```python
from build123d import *

# Parameters (mm, degrees)
BOSS_EXTRUDE1_DEPTH = 5.842
FILLET1_R           = 3.175


with BuildPart() as part:
    # Sketch1 → Boss-Extrude1 (new body)
    with BuildSketch(Plane(origin=(0, 0, 0), x_dir=(1, 0, 0), z_dir=(0, 1, 0))):
        Polygon((25.4, -34.925), (17.895454545, -34.925), (6.35, -19.05), (-6.35, -19.05), (-17.895454545, -34.925), (-25.4, -34.925), (-25.4, -31.75), (-31.242, -31.75), (-31.242, -19.05), (-25.4, -19.05), (-25.4, -14.4526), (-19.05, -14.4526), (-19.05, -15.748), (-15.875, -15.748), (-15.875, -14.4526), (-11.692, -14.4526), (-11.692, -10.9474), (-15.875, -10.9474), (-15.875, -9.652), (-19.05, -9.652), (-19.05, -10.9474), (-25.4, -10.9474), (-25.4, -6.35), (-31.242, -6.35), (-31.242, 6.35), (-25.4, 6.35), (-25.4, 10.9474), (-19.05, 10.9474), (-19.05, 9.652), (-15.875, 9.652), (-15.875, 10.9474), (-11.692, 10.9474), (-11.692, 14.4526), (-15.875, 14.4526), (-15.875, 15.748), (-19.05, 15.748), (-19.05, 14.4526), (-25.4, 14.4526), (-25.4, 19.05), (-31.242, 19.05), (-31.242, 31.75), (-25.4, 31.75), (-25.4, 34.925), (-17.895454545, 34.925), (-6.35, 19.05), (6.35, 19.05), (17.895454545, 34.925), (25.4, 34.925), (25.4, 31.75), (31.242, 31.75), (31.242, 19.05), (25.4, 19.05), (25.4, 14.4526), (19.05, 14.4526), (19.05, 15.748), (15.875, 15.748), (15.875, 14.4526), (11.692, 14.4526), (11.692, 10.9474), (15.875, 10.9474), (15.875, 9.652), (19.05, 9.652), (19.05, 10.9474), (25.4, 10.9474), (25.4, 6.35), (31.242, 6.35), (31.242, -6.35), (25.4, -6.35), (25.4, -10.9474), (19.05, -10.9474), (19.05, -9.652), (15.875, -9.652), (15.875, -10.9474), (11.692, -10.9474), (11.692, -14.4526), (15.875, -14.4526), (15.875, -15.748), (19.05, -15.748), (19.05, -14.4526), (25.4, -14.4526), (25.4, -19.05), (31.242, -19.05), (31.242, -31.75), (25.4, -31.75), align=None)
    extrude(amount=BOSS_EXTRUDE1_DEPTH)

    # Fillet1
    fillet1_edges = [part.edges().sort_by_distance(p)[0] for p in [
        (-17.895454545, 2.921, -34.925),
        (-6.35, 2.921, -19.05),
        (6.35, 2.921, -19.05),
        (17.895454545, 2.921, -34.925),
        (17.895454545, 2.921, 34.925),
        (6.35, 2.921, 19.05),
        (-6.35, 2.921, 19.05),
        (-17.895454545, 2.921, 34.925),
    ]]
    fillet(fillet1_edges, radius=FILLET1_R)


solid = part.part
```
CAD build for the part. Positions are in the model's coordinates, mm. A direction names the side the tool comes from. Round coordinates to 2 decimals unless told otherwise and drop trailing zeros. Order: outer loops, then holes, each group sorted by start corner. A loop starts at its lowest first (then second) coordinate and runs counter-clockwise, first axis right, second up. Notation, with made-up numbers: (77.5, 54.25) -> (121.5, 54.25) arc R25 ccw to (121.5, 89.25) -> close; hole circle Ø11 at (13, 57.5). An arc over 180 degrees is marked (long way). One line per question, with ' | ' between items.
Q1. Probe probe 1 along Z at (x, y) = (28, 4.85); probe 2 along X at (y, z) = (3.1, -14.5) (3 decimals); probe 3 along Z at (x, y) = (-20.5, 2.4) (3 decimals). List the from-to ranges inside material, lowest first.
Completed:
probe 1: z = -31.75 to -19.05, -6.35 to 6.35, 19.05 to 31.75 | probe 2: x = -25.4 to -19.05, -15.875 to 15.875, 19.05 to 25.4 | probe 3: z = -34.925 to -14.453, -10.947 to 10.947, 14.453 to 34.925
Q2. Drop flat-ended pins along their axis: pin 1 (1.8 mm diameter, centred on x = -27, y = 2, fed in from +Z); pin 2 (1.6 mm diameter, centred on x = -17.5, y = 2, fed in from -Z); pin 3 (2.5 mm diameter, centred on x = -17.5, y = 2.5, fed in from +Z). Give the stop position or say it passes through.
Completed:
pin 1: stops at z = 31.75 | pin 2: stops at z = -34.68 | pin 3: stops at z = 34.83
Q3. Slice it at A-A (x = -22.5). Write the cut outline in (y, z) (3 decimals).
Completed:
outline: (0, -34.925) -> (5.842, -34.925) -> (5.842, -14.453) -> (0, -14.453) -> close; (0, -10.947) -> (5.842, -10.947) -> (5.842, 10.947) -> (0, 10.947) -> close; (0, 14.453) -> (5.842, 14.453) -> (5.842, 34.925) -> (0, 34.925) -> close
Q4. Which spindle directions (+Z, -Z, +X, -X, +Y, -Y) get a long thin tool onto all of the face, cutting with end or side? Do faces 4 (the flat face through (-17, 3, 9.652)), 5 (the flat face through (14, 3, -10.947)), 6 (the flat face through (12.19, 2.88, 27.08)). Say none if no direction does.
Completed:
face 4: +Y, -Y | face 5: +X, +Y, -Y | face 6: +Z, +Y, -Y
Q5. Two-plate mould, pull along Z, no slides. Class faces 1 (the flat face through (31.242, 3, 25)), 2 (the flat face through (0, 3, 19.05)), 3 (the flat face through (-28, 3, 6.35)): released by +Z, released by -Z, zero draft, split by the parting line, or undercut.
Completed:
face 1: zero draft | face 2: released by +Z | face 3: undercut
Q6. Slice it at D-D (z = -13.5). Write the cut outline in (x, y).
Completed:
outline: (-11.69, 0) -> (11.69, 0) -> (11.69, 5.84) -> (-11.69, 5.84) -> close
Q7. Slice it at C-C (x = -14.5). Write the cut outline in (y, z).
Completed:
outline: (0, -30.26) -> (5.84, -30.26) -> (5.84, -14.45) -> (0, -14.45) -> close; (0, -10.95) -> (5.84, -10.95) -> (5.84, 10.95) -> (0, 10.95) -> close; (0, 14.45) -> (5.84, 14.45) -> (5.84, 30.26) -> (0, 30.26) -> close
Q8. Slice it at B-B (z = 29). Write the cut outline in (x, y).
Completed:
outline: (-31.24, 0) -> (-13.59, 0) -> (-13.59, 5.84) -> (-31.24, 5.84) -> close; (13.59, 0) -> (31.24, 0) -> (31.24, 5.84) -> (13.59, 5.84) -> close
